Check sheet for the drawn part. Datum: minimum x, y, z corner. Units: mm. Round coordinates to 2 decimals unless told otherwise and drop trailing zeros. Order: outer loops, then holes, each group sorted by start corner. A loop starts at its lowest first (then second) coordinate and runs counter-clockwise, first axis right, second up. Notation, with made-up numbers: (-30.5, -37) - (11.5, -37) arc R18 cw to (11.5, -17) - close; hole circle Ø9 at (58, -2). An arc over 180 degrees is marked (long way). Write each question's results on one line, items separated by ' | '.
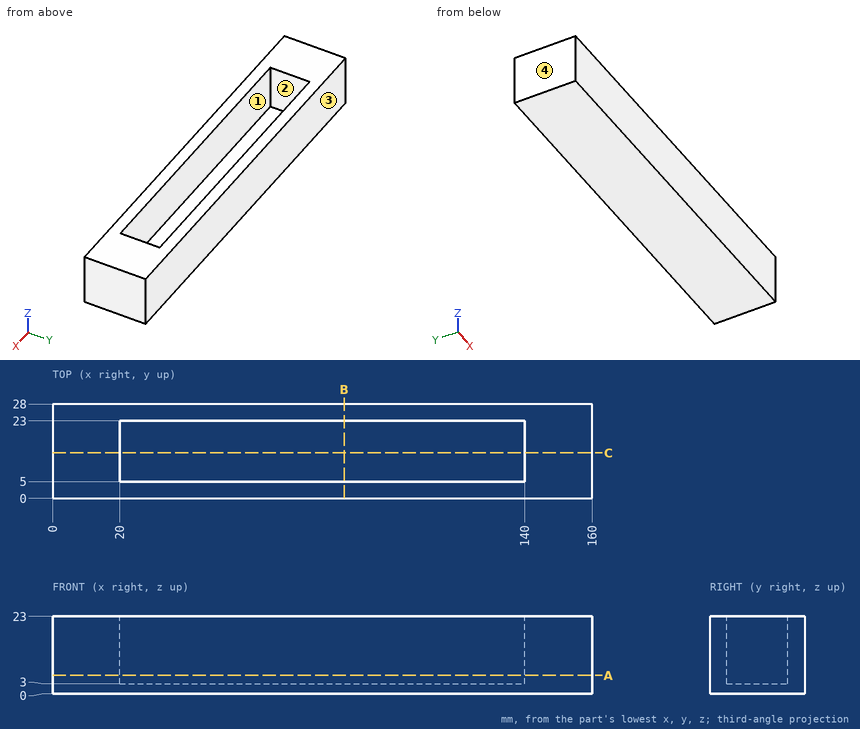
(1) Draft check along Y on the marked faces 1, 2, 3 and 4. Enter one of: released by +Y, released by -Y, zero draft, split by the parting line, or undercut.
Answers follow:
face 1: undercut | face 2: undercut | face 3: released by +Y | face 4: zero draft
(2) Section check C-C (y = 13.5). Record the cut outline in (x, z).
Answers follow:
outline: (0, 0) - (160, 0) - (160, 23) - (140, 23) - (140, 3) - (20, 3) - (20, 23) - (0, 23) - close
(3) Section check B-B (x = 86.5). Record the cut outline in (y, z), then the cut area to 3 significant figures.
Answers follow:
outline: (0, 0) - (28, 0) - (28, 23) - (23, 23) - (23, 3) - (5, 3) - (5, 23) - (0, 23) - close | area: 284 mm²
(4) Depth check by flat-ended pin: pin 1 Ø2 at (x, y) = (111, 7.5) entering from +Z. Enter the tip coordinate at first touch or a pass-through.
Answers follow:
pin 1: z = 3
(5) Material ranges on line 1 (Y direction, x = 83, z = 6.75); line 2 (X direction, y = 16, z = 20.5); line 3 (Z direction, x = 115, y = 15.25), recorded low to high.
Answers follow:
line 1: 0 to 5, 23 to 28 | line 2: 0 to 20, 140 to 160 | line 3: 0 to 3
(6) Section check A-A (z = 5.5). Record the cut outline in (x, y).
Answers follow:
outline: (0, 0) - (160, 0) - (160, 28) - (0, 28) - close; hole (20, 5) - (140, 5) - (140, 23) - (20, 23) - close
